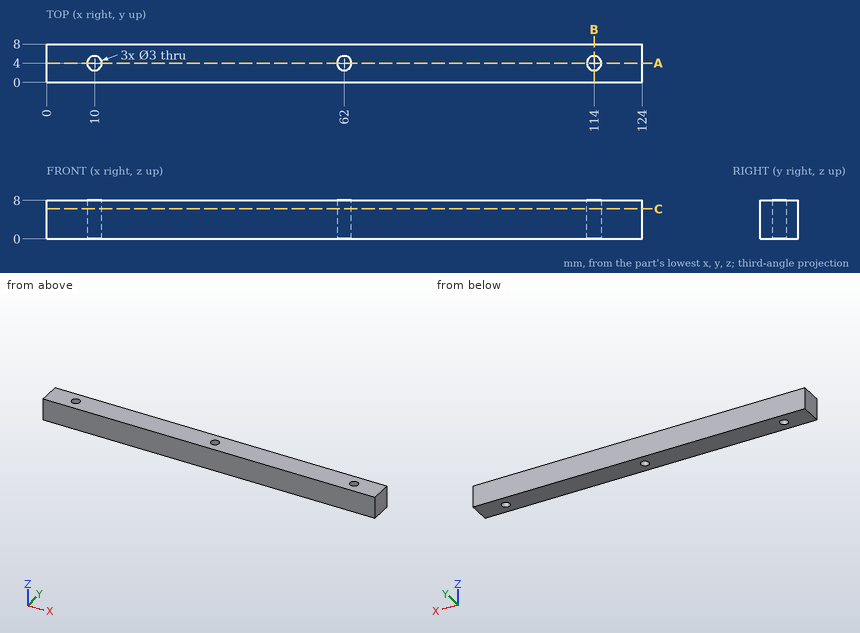
Part print with two shaded views. Sizes in mm from the minimum x, y, z corner. Coordinates: 2 decimals unless noted, no trailing zeros. Write each loop counter-clockwise with the first axis right and the second up, starting at its lowest first coordinate (ties: lowest second). Pieces come first, ordered by that corner, then holes. Notation, with made-up numbers: (89.5, -23.75) -> (118.5, -23.75) arc R33 ccw to (118.5, 10.25) -> close; hole circle Ø4 at (82, 12). An arc over 180 degrees is marked (long way). Return JSON: item names as keys, results as strings. Group by question number.
Q1. Drill centre lines: line 1 (X direction, y = 4.25, z = 2.25); line 2 (Y direction, x = 114, z = 3.25); line 3 (X direction, y = 3.25, z = 6.5). Where is each one in solid material? Low to high.
Q2. Cut at A-A, the plane y = 4. Give the cut face in (x, z), then the cut area to 3 significant figures.
Q3. Cut at B-B, the plane x = 114. Give the cut face in (y, z).
Q4. Cut at C-C, the plane z = 6.25. Give the cut face in (x, y), then the cut area to 3 significant figures.
Returned:
{
 "1": {"line 1": "x = 0 to 8.52, 11.48 to 60.52, 63.48 to 112.52, 115.48 to 124", "line 2": "y = 0 to 2.5, 5.5 to 8", "line 3": "x = 0 to 8.7, 11.3 to 60.7, 63.3 to 112.7, 115.3 to 124"},
 "2": {"outline": "(0, 0) -> (8.5, 0) -> (8.5, 8) -> (0, 8) -> close; (11.5, 0) -> (60.5, 0) -> (60.5, 8) -> (11.5, 8) -> close; (63.5, 0) -> (112.5, 0) -> (112.5, 8) -> (63.5, 8) -> close; (115.5, 0) -> (124, 0) -> (124, 8) -> (115.5, 8) -> close", "area": "920 mm2"},
 "3": {"outline": "(0, 0) -> (2.5, 0) -> (2.5, 8) -> (0, 8) -> close; (5.5, 0) -> (8, 0) -> (8, 8) -> (5.5, 8) -> close"},
 "4": {"outline": "(0, 0) -> (124, 0) -> (124, 8) -> (0, 8) -> close; hole circle Ø3 at (10, 4); hole circle Ø3 at (62, 4); hole circle Ø3 at (114, 4)", "area": "971 mm2"}
}
